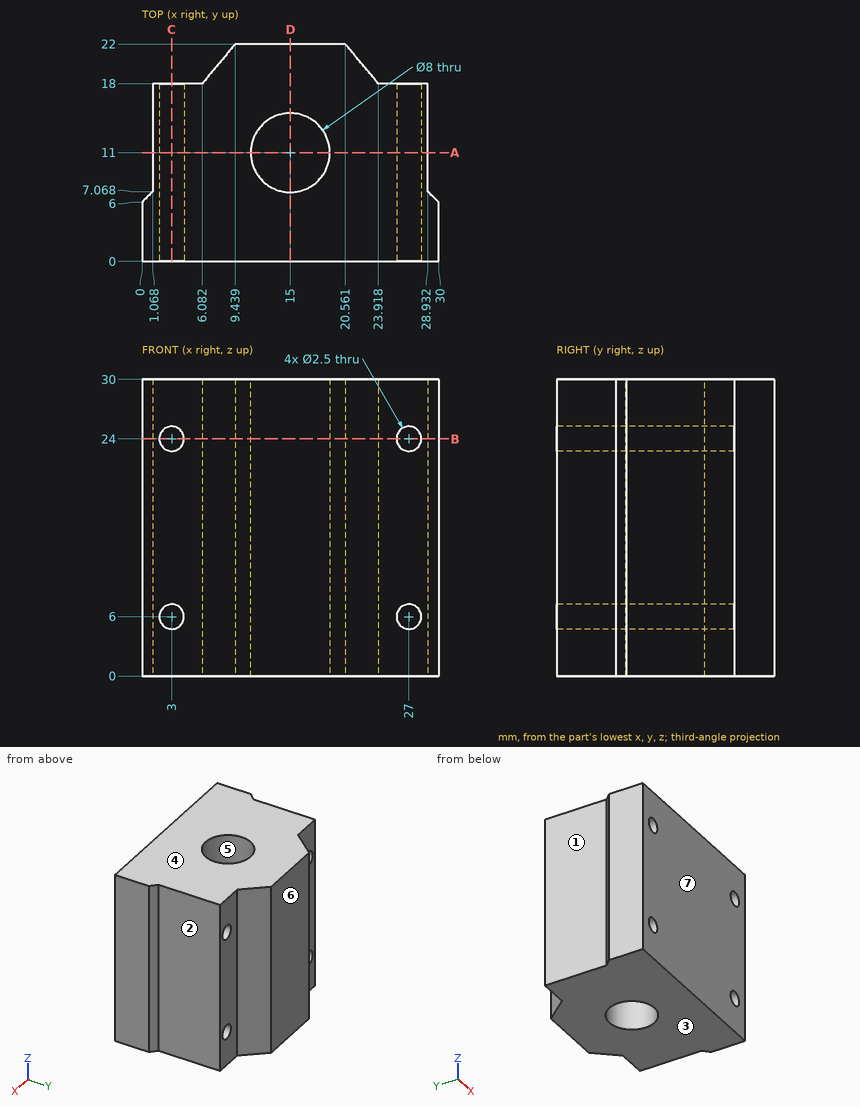
Geometry: see drawing. Coordinates: mm, zero at the bounding-box minimum. A direction names the side the tool comes from. Give positions to 0.01 mm unless a question says otherwise; leave off trailing zeros. Write each loop counter-clockwise with the first axis right and the second up, starting at its lowest first coordinate (ties: lowest second). Pieces come first, ordered by that corner, then holes. Notation, with made-up numbers: M 5,15.5 L 31,15.5 A12 ccw 31,33.5 Z; hole C 75,49 d7. An arc over 180 degrees is marked long. Return JSON: item names as keys, results as strings. Group by question number.
1) Cut plane A-A, the plane y = 11. Output: boundary loops of the cut face in (x, z).
2) Cut plane B-B, the plane z = 24. Output: boundary loops of the cut face in (x, y).
3) Cut plane C-C, the plane x = 3. Output: boundary loops of the cut face in (y, z), then the cut area to 3 significant figures.
4) First-contact query: pin 1 Ø3.5 at (y, z) = (13, 19) entering from +X; pin 2 Ø8.5 at (y, z) = (10.5, 20) entering from -X; pin 3 Ø3 at (y, z) = (11, 14) entering from -X. Flat tips, straight axial feed; report the tip coordinate or a pass-through.
5) Cut plane D-D, the plane x = 15. Output: boundary loops of the cut face in (y, z).
6) Set-up query: the marked faces 1, 2 and 3. Return all of +Z, -Z, +X, -X, +Y, -Y with unobstructed straight access to the full face (end or side cutting, diameter ignored); none if empty.
7) Draft query along Y for the marked faces 4, 5, 6 and 7. Return one class per face: released by +Y, released by -Y, zero draft, split by the parting line, or undercut.
8) Ray query, L1, parallel to Z at x = 3, y = 12.75; L2, parallel to X at y = 5.5, z = 6; L3, parallel to Y at x = 14.75, z = 10.5. Return the intervals inside material, ascending.
Data:
{
 "1": {"outline": "M 1.07,0 L 11,0 L 11,30 L 1.07,30 Z; M 19,0 L 28.93,0 L 28.93,30 L 19,30 Z; hole C 3,6 d2.5; hole C 3,24 d2.5; hole C 27,6 d2.5; hole C 27,24 d2.5"},
 "2": {"outline": "M 0,0 L 1.75,0 L 1.75,18 L 1.07,18 L 1.07,7.07 L 0,6 Z; M 4.25,0 L 25.75,0 L 25.75,18 L 23.92,18 L 20.56,22 L 9.44,22 L 6.08,18 L 4.25,18 Z; M 28.25,0 L 30,0 L 30,6 L 28.93,7.07 L 28.93,18 L 28.25,18 Z; hole C 15,11 d8"},
 "3": {"outline": "M 0,0 L 18,0 L 18,4.75 L 0,4.75 Z; M 0,7.25 L 18,7.25 L 18,22.75 L 0,22.75 Z; M 0,25.25 L 18,25.25 L 18,30 L 0,30 Z", "area": "450 mm²"},
 "4": {"pin 1": "stops at x = 28.93", "pin 2": "stops at x = 0.25", "pin 3": "stops at x = 1.07"},
 "5": {"outline": "M 0,0 L 7,0 L 7,30 L 0,30 Z; M 15,0 L 22,0 L 22,30 L 15,30 Z"},
 "6": {"face 1": "+Z, -Z, -X, +Y", "face 2": "+Z, -Z, +X, +Y", "face 3": "-Z, +X, -X, +Y, -Y"},
 "7": {"face 4": "zero draft", "face 5": "undercut", "face 6": "released by +Y", "face 7": "released by -Y"},
 "8": {"L1": "z = 0 to 4.75, 7.25 to 22.75, 25.25 to 30", "L2": "x = 0 to 1.75, 4.25 to 25.75, 28.25 to 30", "L3": "y = 0 to 7.01, 14.99 to 22"}
}
